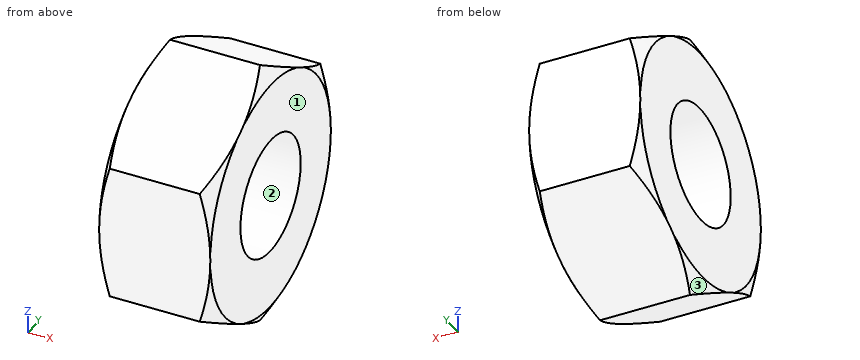
from build123d import *

# Parameters (mm, degrees)
SKETCH1_R      = 4.25
EXTRUDE1_DEPTH = 4


# Read off the part's stored shape, not the designer's step: Cut-Extrude1
with BuildPart() as part:
    # Sketch1 → Extrude1 (new, symmetric)
    with BuildSketch(Plane(origin=(0, 0, 0), x_dir=(0, 0, -1), z_dir=(1, 0, 0))):
        Polygon((9.814954576, 0), (4.907477288, 8.5), (-4.907477288, 8.5), (-9.814954576, 0), (-4.907477288, -8.5), (4.907477288, -8.5), align=None)
        Circle(SKETCH1_R, mode=Mode.SUBTRACT)
    extrude(amount=EXTRUDE1_DEPTH, both=True)

    # Cut-Extrude1 outline → Cut-Extrude1 (revolve, cut)
    with BuildSketch(Plane.YX):
        Polygon((9.81495458, 4.000000073), (8.499999937, 4.000000073), (9.81495458, 3.240810619), align=None)
    cut_extrude1 = revolve(axis=Axis((0, 0, 0), (1, 0, 0)), mode=Mode.SUBTRACT)

    # Mirror1: Cut-Extrude1 across plane
    add(cut_extrude1.mirror(Plane(origin=(0, 0, 0), x_dir=(0, 0, 1), z_dir=(1, 0, 0))), mode=Mode.SUBTRACT)


solid = part.part
Read the model definition and answer for the solid it produces. Units are mm, in the model's axes. Face numbers are marked on the shaded views. Coordinates: 2 decimals unless noted, no trailing zeros. Write each loop counter-clockwise with the first axis right and the second up, starting at its lowest first coordinate (ties: lowest second). Pieces come first, ordered by that corner, then holes. Notation, with made-up numbers: (-20.5, 44) - (3.5, 44) arc R26 cw to (3.5, 70) - close; hole circle Ø9 at (66.25, 87.5). An arc over 180 degrees is marked (long way). One line per question, with ' | ' between items.
Q1. Each of these flat-tipped pins is pushed along its axis until it touches: P1, Ø1, axis at x = -1.5, y = 5, coming from the -Z side; P2, Ø3, axis at x = 0, z = -6, coming from the -Y side. Where does it stop, or does it pass through?
Result set:
P1: z = -7.22 | P2: y = -8.5
Q2. Find section A-A, the plane x = 0.25. Write down the section's boundary in (y, z), plus the area to 3 significant figures.
Result set:
outline: (-8.5, -4.91) - (0, -9.81) - (8.5, -4.91) - (8.5, 4.91) - (0, 9.81) - (-8.5, 4.91) - close; hole circle Ø8.5 at (0, 0) | area: 194 mm^2
Q3. Determine the mould class of the marked faces 1, 2 and 3 for opening direction Y: +Y half, -Y half, draft (parallel to the pull), parting line (faces both ways), or undercut.
Result set:
face 1: draft | face 2: undercut | face 3: parting line
Q4. Find section B-B, the plane x = -3.5. Write down the section's boundary in (y, z).
Result set:
outline: (-8.5, -3.93) arc R9.37 ccw to (-7.66, -5.39) - (-0.84, -9.33) arc R9.37 ccw to (0.84, -9.33) - (7.66, -5.39) arc R9.37 ccw to (8.5, -3.93) - (8.5, 3.93) arc R9.37 ccw to (7.66, 5.39) - (0.84, 9.33) arc R9.37 ccw to (-0.84, 9.33) - (-7.66, 5.39) arc R9.37 ccw to (-8.5, 3.93) - close; hole circle Ø8.5 at (0, 0)
Q5. Consider L1, parallel to Y at x = 2, z = 0; L2, parallel to Y at x = 0, z = -2.75; L3, parallel to Z at x = 3, y = 2.25. Determine where each line is inside the solid, lowest interval first. Write a range as [from, to].
Result set:
L1: [-8.5, -4.25], [4.25, 8.5] | L2: [-8.5, -3.24], [3.24, 8.5] | L3: [-8.52, -3.61], [3.61, 8.52]
